from build123d import *

# Parameters (mm, degrees)
SKETCH1_R           = 2.5
BOSS_EXTRUDE1_DEPTH = 8
SKETCH2_R           = 5.5
BOSS_EXTRUDE2_DEPTH = 0.5
BOSS_EXTRUDE3_DEPTH = 3
CHAMFER3_SIZE       = 0.5


with BuildPart() as part:
    # Sketch1 → Boss-Extrude1 (new body)
    with BuildSketch(Plane.XY):
        Circle(SKETCH1_R)
    extrude(amount=BOSS_EXTRUDE1_DEPTH)

    # Sketch2 → Boss-Extrude2 (add)
    with BuildSketch(Plane(origin=(0, 0, 0), x_dir=(-1, 0, 0), z_dir=(0, 0, -1))):
        Circle(SKETCH2_R)
    extrude(amount=BOSS_EXTRUDE2_DEPTH)

    # Sketch3 → Boss-Extrude3 (add)
    with BuildSketch(Plane(origin=(0, 0, -0.5), x_dir=(-1, 0, 0), z_dir=(0, 0, -1))):
        Polygon((4.041451884, 0), (2.020725942, 3.5), (-2.020725942, 3.5), (-4.041451884, 0), (-2.020725942, -3.5), (2.020725942, -3.5), align=None)
    extrude(amount=BOSS_EXTRUDE3_DEPTH)

    # Chamfer3
    chamfer3_edges = [part.edges().sort_by_distance(p)[0] for p in [
        (-2.5, 0, 8),
    ]]
    chamfer(chamfer3_edges, length=CHAMFER3_SIZE)


solid = part.part
Geometry check sheet. Reference: the model listing, model coordinates, mm. A direction names the side the tool comes from. Round coordinates to 2 decimals unless told otherwise and drop trailing zeros. Loops run counter-clockwise (first coordinate to the right, second up) from the corner with the lowest first, then second, coordinate; pieces in that order, holes last.
Item 1: Cross-section at B-B on z = -2.5. Record the boundary of the cut face in (x, y).
Item 2: Thickness scan on line 1 (Z direction, x = 3, y = -2); line 2 (Y direction, x = 0, z = -1.25); line 3 (X direction, y = 1.5, z = 2). Record the ranges inside material, lowest first.
Item 3: Access from +Z, -Z, +X, -X, +Y, -Y to the whole of each face (thin tool, end or side, straight path). Record for faces 1 (the cylindrical face through (-0.54, -2.44, 3.7)), 2 (the flat face through (3.045, -1.726, -1.979)), 3 (the flat face through (3, 1.8, -2)).
Item 4: Cross-section at D-D on x = -3. Record the boundary of the cut face in (y, z).
Item 5: Cross-section at C-C on y = -2.75. Record the boundary of the cut face in (x, z), then the cut area to 3 significant figures.
Item 6: Gauge pin test, flat ends, axial feed: pin 1 (1.5 mm diameter, centred on x = -0.5, z = 2.5, fed in from +Y); pin 2 (1.5 mm diameter, centred on x = -0.5, z = -1.5, fed in from -Y); pin 3 (5 mm diameter, centred on y = 4, z = -0.5, fed in from +X). Record the tip position at first contact, or that the pin passes through.
Item 7: Cross-section at A-A on x = 0. Record the boundary of the cut face in (y, z).
Answer sheet:
1. outline: (-4.04, 0) - (-2.02, -3.5) - (2.02, -3.5) - (4.04, 0) - (2.02, 3.5) - (-2.02, 3.5) - close
2. line 1: z = -0.5 to 0
2. line 2: y = -3.5 to 3.5
2. line 3: x = -2 to 2
3. face 1: +Z
3. face 2: -Z, +X, -Y
3. face 3: -Z, +X, +Y
4. outline: (-4.61, -0.5) - (-1.8, -0.5) - (-1.8, -3.5) - (1.8, -3.5) - (1.8, -0.5) - (4.61, -0.5) - (4.61, 0) - (-4.61, 0) - close
5. outline: (-4.76, -0.5) - (-2.45, -0.5) - (-2.45, -3.5) - (2.45, -3.5) - (2.45, -0.5) - (4.76, -0.5) - (4.76, 0) - (-4.76, 0) - close
5. area: 19.5 mm2
6. pin 1: stops at y = 2.5
6. pin 2: stops at y = -3.5
6. pin 3: stops at x = 5.29
7. outline: (-5.5, -0.5) - (-3.5, -0.5) - (-3.5, -3.5) - (3.5, -3.5) - (3.5, -0.5) - (5.5, -0.5) - (5.5, 0) - (2.5, 0) - (2.5, 7.5) - (2, 8) - (-2, 8) - (-2.5, 7.5) - (-2.5, 0) - (-5.5, 0) - close
